Geometry check sheet. Reference: the model listing, model coordinates, mm. Face numbers are marked on the shaded views. A direction names the side the tool comes from. Round coordinates to 2 decimals unless told otherwise and drop trailing zeros. Write each loop counter-clockwise with the first axis right and the second up, starting at its lowest first coordinate (ties: lowest second). Pieces come first, ordered by that corner, then holes.
Item 1: Cross-section at D-D (x = -101). Enter the section's corners in (y, z), then the cut area to 3 significant figures.
Item 2: Scan lines: probe 1 along Z at (x, y) = (11, 0); probe 2 along Y at (x, z) = (-100, -93); probe 3 along X at (y, z) = (-60, 157). Record each from-to range of solid material in increasing order.
Item 3: Draft check along Z on the marked faces 1, 2 and 3. Enter one of: pulls with the +Z half, pulls with the -Z half, needs draft (parallel to the pull), parting line crosses it, or undercut.
Item 4: Cross-section at C-C (x = -39). Enter the section's corners in (y, z).
Item 5: Depth check by flat-ended pin: P1, Ø3, axis at y = -4, z = -56, coming from the -X side; P2, Ø3, axis at x = -199, y = 56.5, coming from the +Z side; P3, Ø10, axis at y = -45, z = 121, coming from the +X side; P4, Ø7.5, axis at y = -72, z = 106.16, coming from the -X side. Enter the tip coordinate at first touch or a pass-through.
Item 6: Cross-section at A-A (x = -220). Enter the section's corners in (y, z).
Item 7: Cross-section at B-B (y = -60). Enter the section's corners in (x, z), then the cut area to 3 significant figures.
Item 8: Access from +Z, -Z, +X, -X, +Y, -Y to the whole of each face (thin tool, end or side, straight path). Record for the marked faces 4, 5 and 6.
from build123d import *

# Parameters (mm, degrees)
F1_DEPTH        = 40
F2_W            = 300
F2_H            = 200
F3_DEPTH        = 40
F4_W            = 83.487585187
F4_H            = 50
F5_DEPTH        = 60
F7_DEPTH        = 125.001
F8_R            = 10
F10_D           = 12.1
F11_SIZE        = 5
F13_D           = 17.5
F13_CBORE_D     = 31.5
F13_CBORE_DEPTH = 20
F14_SIZE        = 10


with BuildPart() as f1:
    # F0 (on Right) → F1 (new body)
    with BuildSketch(Plane.YZ):
        with BuildLine():
            Line((-100, 106.1599394854), (-100, -106.1599394854))
            Line((-100, -106.1599394854), (100, -106.1599394854))
            Line((100, -106.1599394854), (100, 106.1599394854))
            Line((100, 106.1599394854), (50, 106.1599394854))
            ThreePointArc((50, 106.1599394854), (0, 56.1599394854), (-50, 106.1599394854))
            Line((-50, 106.1599394854), (-100, 106.1599394854))
        make_face()
        with BuildLine():
            ThreePointArc((100, 106.1599394854), (0, 206.1599394854), (-100, 106.1599394854))
            Line((-100, 106.1599394854), (-50, 106.1599394854))
            ThreePointArc((-50, 106.1599394854), (0, 156.1599394854), (50, 106.1599394854))
            Line((50, 106.1599394854), (100, 106.1599394854))
        make_face()
    extrude(amount=F1_DEPTH)

    # F2 (on face) → F3 (join)
    with BuildSketch(Plane(origin=(0, 0, -106.1599394854), x_dir=(1, 0, 0), z_dir=(0, 0, -1))):
        with Locations((-110, 0)):
            Rectangle(F2_W, F2_H)
    extrude(amount=-F3_DEPTH)

    # F4 (on face) → F5 (join)
    with BuildSketch(Plane.XY.offset(-66.1599394854)):
        with Locations((-41.7437925935, 0)):
            Rectangle(F4_W, F4_H)
    extrude(amount=F5_DEPTH)

    # F6 (on face) → F7 (cut, through all)
    with BuildSketch(Plane(origin=(0, 25, 0), x_dir=(-1, 0, 0), z_dir=(0, 1, 0))):
        Polygon((83.487585187, -6.1599394854), (0, -6.1599394854), (83.487585187, -66.1599394854), align=None)
    extrude(amount=-F7_DEPTH, mode=Mode.SUBTRACT)

    # F8
    f8_edges = [f1.edges().sort_by_distance(p)[0] for p in [
        (0, 62.5, -66.159939),
        (0, -62.5, -66.159939),
    ]]
    fillet(f8_edges, radius=F8_R)

    # F10 (through all)
    with Locations(Plane(origin=(0, 0, 0), x_dir=(0, -1, 0), z_dir=(-1, 0, 0))):
        with Locations((0, 178.1599394854), (-72, 106.1599394854), (0, 34.1599394854), (72, 106.1599394854)):
            Hole(F10_D / 2)

    # F11
    f11_edges = [f1.edges().sort_by_distance(p)[0] for p in [
        (0, 50, 106.159939),
        (40, 50, 106.159939),
    ]]
    chamfer(f11_edges, length=F11_SIZE)

    # F13 (through all)
    with Locations(Plane.XY.offset(-66.1599394854)):
        with Locations((-220, 60), (-220, -60), (-100, 60), (-100, -60)):
            CounterBoreHole(F13_D / 2, F13_CBORE_D / 2, F13_CBORE_DEPTH)

    # F14
    f14_edges = [f1.edges().sort_by_distance(p)[0] for p in [
        (-260, 100, -86.159939),
        (-260, -100, -86.159939),
    ]]
    chamfer(f14_edges, length=F14_SIZE)


solid = f1.part
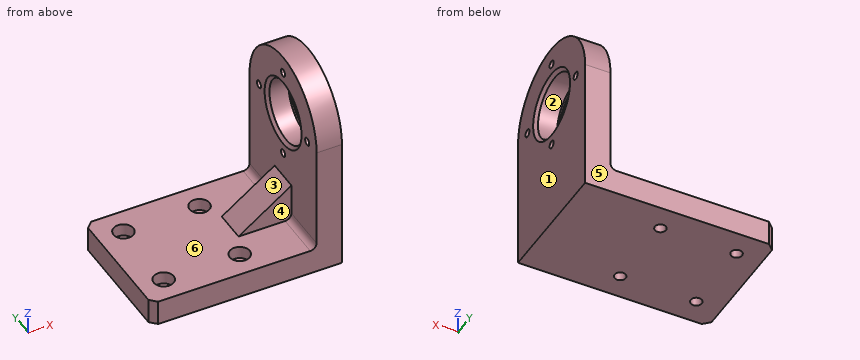
Resolved:
1. outline: (-100, -106.16) - (-68.69, -106.16) - (-68.69, -86.16) - (-75.72, -86.16) - (-75.72, -66.16) - (-100, -66.16) - close; (-51.31, -106.16) - (51.31, -106.16) - (51.31, -86.16) - (44.28, -86.16) - (44.28, -66.16) - (-44.28, -66.16) - (-44.28, -86.16) - (-51.31, -86.16) - close; (68.69, -106.16) - (100, -106.16) - (100, -66.16) - (75.72, -66.16) - (75.72, -86.16) - (68.69, -86.16) - close
1. area: 6,050 mm2
2. probe 1: z = -106.16 to 28.11, 40.21 to 56.16, 156.16 to 172.11, 184.21 to 206.16
2. probe 2: y = -100 to -68.75, -51.25 to 51.25, 68.75 to 100
2. probe 3: x = 0 to 40
3. face 1: needs draft
3. face 2: undercut
3. face 3: pulls with the +Z half
4. outline: (-100, -106.16) - (100, -106.16) - (100, -66.16) - (25, -66.16) - (25, -34.19) - (-25, -34.19) - (-25, -66.16) - (-100, -66.16) - close
5. P1: stops at x = -71.44
5. P2: stops at z = -66.16
5. P3: stops at x = 37.38
5. P4: passes through
6. outline: (-100, -106.16) - (-68.75, -106.16) - (-68.75, -86.16) - (-75.75, -86.16) - (-75.75, -66.16) - (-100, -66.16) - close; (-51.25, -106.16) - (51.25, -106.16) - (51.25, -86.16) - (44.25, -86.16) - (44.25, -66.16) - (-44.25, -66.16) - (-44.25, -86.16) - (-51.25, -86.16) - close; (68.75, -106.16) - (100, -106.16) - (100, -66.16) - (75.75, -66.16) - (75.75, -86.16) - (68.75, -86.16) - close
7. outline: (-260, -106.16) - (-228.75, -106.16) - (-228.75, -86.16) - (-235.75, -86.16) - (-235.75, -66.16) - (-260, -66.16) - close; (-211.25, -106.16) - (-108.75, -106.16) - (-108.75, -86.16) - (-115.75, -86.16) - (-115.75, -66.16) - (-204.25, -66.16) - (-204.25, -86.16) - (-211.25, -86.16) - close; (-91.25, -106.16) - (40, -106.16) - (40, 186.16) - (0, 186.16) - (0, -56.16) arc R10 cw to (-10, -66.16) - (-84.25, -66.16) - (-84.25, -86.16) - (-91.25, -86.16) - close
7. area: 20,200 mm2
8. face 4: +Z, -X, -Y
8. face 5: +Z, -Z, +X, -X, +Y
8. face 6: +Z, -X
